Design review of the part built by this model. Coordinates are the model's own, in mm. A direction names the side the tool comes from. Round coordinates to 2 decimals unless told otherwise and drop trailing zeros. Loops run counter-clockwise (first coordinate to the right, second up) from the corner with the lowest first, then second, coordinate; pieces in that order, holes last. Notation, with made-up numbers: (-11.5, 47.5) -> (41.5, 47.5) arc R26 cw to (41.5, 72.5) -> close; hole circle Ø6 at (31.5, 10.25). An arc over 180 degrees is marked (long way). Use a Markdown table: item, result. Add a question column.
from build123d import *

# Parameters (mm, degrees)
SKETCH1_R                        = 113
BOSS_EXTRUDE1_DEPTH              = 74
SKETCH2_R                        = 129
SKETCH2_R_2                      = 70
CUT_EXTRUDE1_DEPTH               = 20
SKETCH3_W                        = 90
SKETCH3_H                        = 77.119146837
SKETCH6_W                        = 6
SKETCH6_H                        = 11.156401333
CHAMFER1_SIZE                    = 1
SKETCH9_W                        = 55
SKETCH9_H                        = 44.304211173
CUT_EXTRUDE2_DEPTH               = 122.5
F_1_2_14_NPSM_TAPPED_HOLE1_D     = 18.9738
F_1_2_14_NPSM_TAPPED_HOLE1_DEPTH = 100
F_1_2_14_NPSM_TAPPED_HOLE1_TIP   = 5.700304607
CHAMFER2_SIZE                    = 2
SKETCH13_R                       = 8.5
CUT_EXTRUDE3_DEPTH               = 59.0000001
CIRPATTERN3_COUNT                = 4
FILLET1_R                        = 2
FILLET2_R                        = 3


with BuildPart() as part:
    # Sketch1 → Boss-Extrude1 (new body, symmetric)
    with BuildSketch(Plane.XY):
        Circle(SKETCH1_R)
    extrude(amount=BOSS_EXTRUDE1_DEPTH, both=True)

    # Sketch2 → Cut-Extrude1 (cut)
    with BuildSketch(Plane(origin=(0, 0, -74), x_dir=(-1, 0, 0), z_dir=(0, 0, -1))):
        Circle(SKETCH2_R)
        Circle(SKETCH2_R_2, mode=Mode.SUBTRACT)
    extrude(amount=-CUT_EXTRUDE1_DEPTH, mode=Mode.SUBTRACT)

    # Sketch3 → Cut-Revolve1 (revolve, cut)
    with BuildSketch(Plane(origin=(0, 0, 0), x_dir=(0, 0, -1), z_dir=(1, 0, 0))):
        with Locations((-29, 116.059573419)):
            Rectangle(SKETCH3_W, SKETCH3_H)
    revolve(axis=Axis((0, 0, 0), (0, 0, 1)), mode=Mode.SUBTRACT)

    # Sketch6 → Cut-Revolve2 (revolve, cut)
    with BuildSketch(Plane(origin=(0, 0, 0), x_dir=(0, 0, -1), z_dir=(1, 0, 0))):
        with Locations((66, 71.578200667)):
            Rectangle(SKETCH6_W, SKETCH6_H)
    revolve(axis=Axis((0, 0, 0), (0, 0, -1)), mode=Mode.SUBTRACT)

    # Chamfer1
    chamfer1_edges = [part.edges().sort_by_distance(p)[0] for p in [
        (70, 0, -74),
    ]]
    chamfer(chamfer1_edges, length=CHAMFER1_SIZE)

    # Sketch9 → Cut-Extrude2 (cut, symmetric)
    with BuildSketch(Plane.XY):
        with Locations((0, 131.75479716)):
            Rectangle(SKETCH9_W, SKETCH9_H)
    extrude(amount=CUT_EXTRUDE2_DEPTH, both=True, mode=Mode.SUBTRACT)

    # 1/2-14 NPSM Tapped Hole1
    with Locations(Plane(origin=(0, 109.602691573, 0), x_dir=(1, 0, 0), z_dir=(0, 1, 0))):
        with Locations((0, 35)):
            Hole(F_1_2_14_NPSM_TAPPED_HOLE1_D / 2, depth=F_1_2_14_NPSM_TAPPED_HOLE1_DEPTH)
            with Locations((0, 0, -(F_1_2_14_NPSM_TAPPED_HOLE1_DEPTH + F_1_2_14_NPSM_TAPPED_HOLE1_TIP / 2))):  # 118° drill point
                Cone(0, F_1_2_14_NPSM_TAPPED_HOLE1_D / 2, F_1_2_14_NPSM_TAPPED_HOLE1_TIP, mode=Mode.SUBTRACT)

    # Sketch7 → Cut-Revolve3 (revolve, cut)
    with BuildSketch(Plane(origin=(0, 0, 0), x_dir=(0, -1, 0), z_dir=(1, 0, 0))):
        Polygon((-42, -74), (-42, -71), (-44.3, -71), (-44.3, -65.8), (-40.25, -65.8), (-40.25, -57.8), (-45, -57.8), (-45, -46.8), (-40.25, -46.8), (-40.25, -39.8), (-47.55, -39.8), (-47.55, -33.5), (-40.25, -33.5), (-40.25, -27.5), (-42.5, -27.5), (-42.5, 22.5), (-45, 22.5), (-45, 96.107724416), (-36.150119244, 96.107724416), (0, 96.107724416), (0, -74), align=None)
    revolve(axis=Axis((0, 0, 0), (0, 0, 1)), mode=Mode.SUBTRACT)

    # Chamfer2
    chamfer2_edges = [part.edges().sort_by_distance(p)[0] for p in [
        (9.4869, 109.602691573, -35),
    ]]
    chamfer(chamfer2_edges, length=CHAMFER2_SIZE)

    # Sketch13 → Cut-Extrude3 (cut, through all)
    with BuildSketch(Plane.XY.offset(-16)):
        with Locations((-69.296464556, 69.296464556)):
            Circle(SKETCH13_R)
        with Locations((-37.502976372, 90.540194186)):
            Circle(SKETCH13_R)
        with Locations((-90.540194186, 37.502976372)):
            Circle(SKETCH13_R)
    cut_extrude3 = extrude(amount=-CUT_EXTRUDE3_DEPTH, mode=Mode.SUBTRACT)

    # CirPattern3: Cut-Extrude3 ×4 about axis
    cirpattern3_axis = Axis((0, 0, 0), (0, 0, 1))
    for i in range(1, CIRPATTERN3_COUNT):
        add(cut_extrude3.rotate(cirpattern3_axis, i * 360 / CIRPATTERN3_COUNT), mode=Mode.SUBTRACT)

    # Fillet1
    fillet1_edges = [part.edges().sort_by_distance(p)[0] for p in [
        (0, -77.5, -16),
        (0, -113, -16),
        (0, 109.602691573, -16),
    ]]
    fillet(fillet1_edges, radius=FILLET1_R)

    # Fillet2
    fillet2_edges = [part.edges().sort_by_distance(p)[0] for p in [
        (0, -77.5, 74),
    ]]
    fillet(fillet2_edges, radius=FILLET2_R)


solid = part.part
1. To check wall thickness, follow probe 1 along Y at (x, z) = (-72, -24); probe 2 along Z at (x, y) = (62.5, 22); probe 3 along Y at (x, z) = (31.5, -17.5). State the ranges of each line that lie inside material, in increasing order. Write a range as from..to.
2. Consider section A-A on z = -35. Give the number of separate pieces and of enclosed holes in the cut face, plus the area to 3 significant figures.
3. Consider section C-C on z = 0. State the section outline as (x, y) points.
4. Mouldability with a two-part tool opening along Y and no side actions: class faces 1 (the face through (43.247, -9.603, 68.364)), 2 (the face through (1.235, 75.35, -44.406)), 3 (the face through (-64.43, -14.31, -66.04)) as +Y half, -Y half, draft (parallel to the pull), parting line (faces both ways), or undercut.
5. For faces 4 (the face through (38, -16, 27.5)), 5 (the face through (83, 33.58, -34.73)), 6 (the face through (23, -34, 46.8)), 7 (the face through (49, 64, -16)), list the 3-axis set-ups (+Z, -Z, +X, -X, +Y, -Y) from which the entire face can be reached by the end or side of a thin tool; tool diameter is ignored.
6. Insertion check: P1, Ø2, axis at x = -20.5, y = 76.5, coming from the -Z side; P2, Ø5, axis at x = -0.5, z = 0.5, coming from the +Y side; P3, Ø1, axis at x = -83, z = -32.5, coming from the -Y side; P4, Ø10, axis at x = 37.5, y = -90.54, coming from the +Z side. Each pin has a flat end and moves straight along its axis. Give the tip position at first contact, or say it passes through.
Verdict:
| question | item | result |
|---|---|---|
| 1 | probe 1 | y = -87.09..-77.36, -61.24..61.24, 77.36..87.09 |
| 1 | probe 2 | z = -74..-69, -63..74 |
| 1 | probe 3 | y = -108.45..-96.56, -84.52..-28.53, 28.53..84.52, 96.56..108.45 |
| 2 | separate pieces | 1 |
| 2 | enclosed holes | 12 |
| 2 | area | 29,700 mm² |
| 3 | outline | circle Ø155 at (0, 0); hole circle Ø85 at (0, 0) |
| 4 | face 1 | undercut |
| 4 | face 2 | draft |
| 4 | face 3 | parting line |
| 5 | face 4 | -Z |
| 5 | face 5 | +Z, -Z |
| 5 | face 6 | none |
| 5 | face 7 | +Z |
| 6 | P1 | stops at z = -54 |
| 6 | P2 | stops at y = 77.5 |
| 6 | P3 | stops at y = -77.22 |
| 6 | P4 | passes through |
